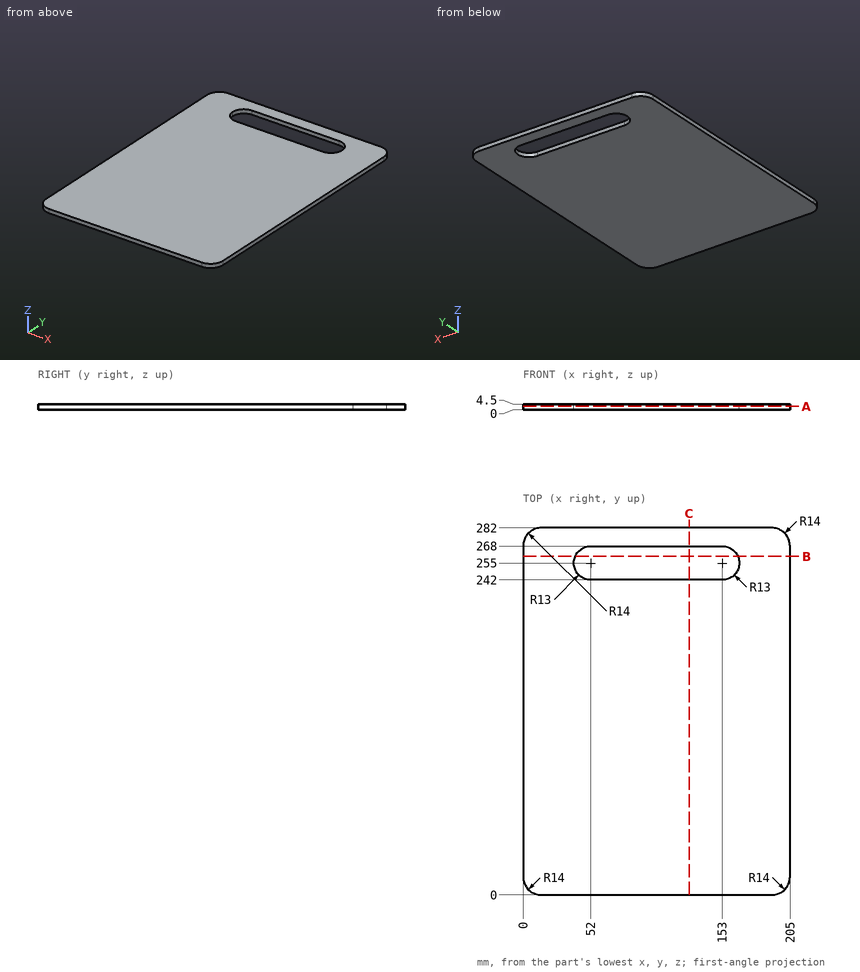
Could you check a few things on this drawing? It's one solid part, dimensions in mm from its lowest x, y, z. Round coordinates to 2 decimals unless told otherwise and drop trailing zeros. Order: outer loops, then holes, each group sorted by start corner. A loop starts at its lowest first (then second) coordinate and runs counter-clockwise, first axis right, second up. Notation, with made-up numbers: M 14,61 L 64,61 A26 ccw 64,75 Z; hole C -16,-3 d4. An arc over 180 degrees is marked long. One line per item, written item: value.
(1) Imagine slicing it at A-A (z = 2.75). Write out the boundary of the cut face in (x, y), and give its area (3 significant figures).
Ans:
outline: M 0,14 A14 ccw 14,0 L 191,0 A14 ccw 205,14 L 205,268 A14 ccw 191,282 L 14,282 A14 ccw 0,268 Z; hole M 39,255 A13 ccw 52,242 L 153,242 A13 ccw 166,255 A13 ccw 153,268 L 52,268 A13 ccw Z
area: 54,500 mm^2
(2) Imagine slicing it at C-C (x = 127.5). Write out the boundary of the cut face in (y, z).
Ans:
outline: M 0,0 L 242,0 L 242,4.5 L 0,4.5 Z; M 268,0 L 282,0 L 282,4.5 L 268,4.5 Z
(3) Imagine slicing it at B-B (y = 260). Write out the boundary of the cut face in (x, z), and give its area (3 significant figures).
Ans:
outline: M 0,0 L 40,0 L 40,4.5 L 0,4.5 Z; M 165,0 L 205,0 L 205,4.5 L 165,4.5 Z
area: 360 mm^2
(4) I need wall thicknesses on line 1 along Y through (x, z) = (117, 1.75); line 2 along X through (y, z) = (251.5, 3); line 3 along Y through (x, z) = (48, 3.4). Which ranges of each line are inside material? Lowest first, please. Write a range as from..to.
Ans:
line 1: y = 0..242, 268..282
line 2: x = 0..39.48, 165.52..205
line 3: y = 0..242.63, 267.37..282
